from build123d import *

# Parameters (mm, degrees)
SKETCH1_R                                      = 44.45
BOSS_EXTRUDE1_DEPTH                            = 6.35
SKETCH2_R                                      = 13.5
CUT_EXTRUDE1_DEPTH                             = 65.131856359
CSK_FOR_0_FLAT_HEAD_MACHINE_SCREW1_D           = 1.778
CSK_FOR_0_FLAT_HEAD_MACHINE_SCREW1_CSINK_D     = 3.0226
CSK_FOR_0_FLAT_HEAD_MACHINE_SCREW1_CSINK_ANGLE = 82
CIRPATTERN1_COUNT                              = 8
SKETCH6_W                                      = 12.7
SKETCH6_H                                      = 25.4
BOSS_EXTRUDE2_DEPTH                            = 50.8
FILLET1_R                                      = 12.7
SKETCH7_R                                      = 6.35
CUT_EXTRUDE2_DEPTH                             = 106.111203019


with BuildPart() as part:
    # Sketch1 → Boss-Extrude1 (new, symmetric)
    with BuildSketch(Plane.XY):
        Circle(SKETCH1_R)
    extrude(amount=BOSS_EXTRUDE1_DEPTH, both=True)

    # Sketch2 → Cut-Extrude1 (cut, through all)
    with BuildSketch(Plane.XY.offset(6.35)):
        Circle(SKETCH2_R)
    extrude(amount=-CUT_EXTRUDE1_DEPTH, mode=Mode.SUBTRACT)

    # CSK for #0 Flat Head Machine Screw1 (through all)
    with Locations(Plane(origin=(-0.166965968, 41.999668122, 6.35), x_dir=(1, 0, 0), z_dir=(0, 0, 1))):
        with Locations((0, 0)):
            csk_for_0_flat_head_machine_screw1 = CounterSinkHole(CSK_FOR_0_FLAT_HEAD_MACHINE_SCREW1_D / 2, CSK_FOR_0_FLAT_HEAD_MACHINE_SCREW1_CSINK_D / 2, counter_sink_angle=CSK_FOR_0_FLAT_HEAD_MACHINE_SCREW1_CSINK_ANGLE)

    # CirPattern1: CSK for #0 Flat Head Machine Screw1 ×8 about axis
    cirpattern1_axis = Axis((0, 0, 0), (0, 0, 1))
    for i in range(1, CIRPATTERN1_COUNT):
        add(csk_for_0_flat_head_machine_screw1.rotate(cirpattern1_axis, i * 360 / CIRPATTERN1_COUNT), mode=Mode.SUBTRACT)

    # Sketch6 → Boss-Extrude2 (add)
    with BuildSketch(Plane.XY.offset(6.35)):
        with Locations((-25.4, 0)):
            Rectangle(SKETCH6_W, SKETCH6_H)
        with Locations((25.4, 0)):
            Rectangle(SKETCH6_W, SKETCH6_H)
    extrude(amount=BOSS_EXTRUDE2_DEPTH)

    # Fillet1
    fillet1_edges = [part.edges().sort_by_distance(p)[0] for p in [
        (-25.4, 12.7, 57.15),
        (-25.4, -12.7, 57.15),
        (25.4, -12.7, 57.15),
        (25.4, 12.7, 57.15),
    ]]
    fillet(fillet1_edges, radius=FILLET1_R - 0.0001)  # a hair under: the kernel refuses the full size

    # Sketch7 → Cut-Extrude2 (cut, through all)
    with BuildSketch(Plane(origin=(31.75, 0, 0), x_dir=(0, 0, -1), z_dir=(1, 0, 0))):
        with Locations((-44.45, 0)):
            Circle(SKETCH7_R)
    extrude(amount=-CUT_EXTRUDE2_DEPTH, mode=Mode.SUBTRACT)


solid = part.part
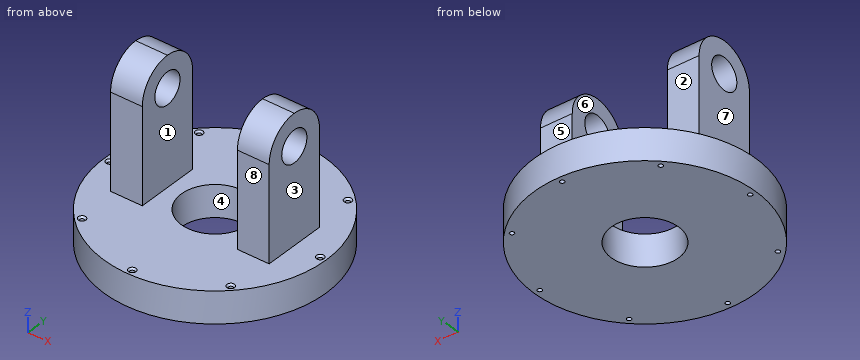
Geometry check sheet. Reference: the model listing, model coordinates, mm. Face numbers are marked on the shaded views. A direction names the side the tool comes from. Coordinates: 2 decimals unless noted, no trailing zeros. Order: outer loops, then holes, each group sorted by start corner. A loop starts at its lowest first (then second) coordinate and runs counter-clockwise, first axis right, second up. Notation, with made-up numbers: (54, 21) -> (108, 21) arc R30 ccw to (108, 46) -> close; hole circle Ø5 at (-6.75, -40). An arc over 180 degrees is marked (long way). Use a Markdown table: item, result. Add a question column.
1. Mould release check, pull along X, two halves, no side actions. Record for the marked faces 1, 2, 3 and 4: pulls with the +X half, pulls with the -X half, needs draft (parallel to the pull), parting line crosses it, or undercut.
2. Set-up check for the marked faces 5, 6, 7 and 8: record each of +Z, -Z, +X, -X, +Y, -Y from which the full face is reachable in a straight line by a thin tool's end or side.
3. Cross-section at D-D (y = 36.5). Enter the section's corners in (x, z), and give its area (3 significant figures).
4. Cross-section at A-A (z = 10). Enter the section's corners in (x, y), and give its area (3 significant figures).
5. Go/stop test with flat-tipped pins: pin 1 Ø2 at (x, y) = (29.58, 29.82) entering from +Z; pin 2 Ø6.5 at (x, z) = (-24, 17) entering from -Y; pin 3 Ø1.5 at (x, z) = (-20, 29) entering from +Y; pin 4 Ø7.5 at (y, z) = (0, 44.45) entering from -X. Record where each tip stops, or that it passes through.
6. Cross-section at C-C (y = 10). Enter the section's corners in (x, z), and give its area (3 significant figures).
7. Cross-section at B-B (x = -9). Enter the section's corners in (y, z).
8. Material ranges on L1, parallel to X at y = 12, z = 44; L2, parallel to Y at x = 0, z = 3.5; L3, parallel to Y at x = 25, z = 44, recorded low to high.
Filled sheet:
| question | item | result |
|---|---|---|
| 1 | face 1 | undercut |
| 1 | face 2 | needs draft |
| 1 | face 3 | pulls with the +X half |
| 1 | face 4 | undercut |
| 2 | face 5 | +Z, +X, -X, +Y |
| 2 | face 6 | +Z, +Y, -Y |
| 2 | face 7 | +Z, -X, +Y, -Y |
| 2 | face 8 | +Z, +X, -X, -Y |
| 3 | outline | (-25.37, -6.35) -> (25.37, -6.35) -> (25.37, 6.35) -> (-25.37, 6.35) -> close |
| 3 | area | 644 mm2 |
| 4 | outline | (-31.75, -12.7) -> (-19.05, -12.7) -> (-19.05, 12.7) -> (-31.75, 12.7) -> close; (19.05, -12.7) -> (31.75, -12.7) -> (31.75, 12.7) -> (19.05, 12.7) -> close |
| 4 | area | 645 mm2 |
| 5 | pin 1 | z = 5.77 |
| 5 | pin 2 | y = -12.7 |
| 5 | pin 3 | y = 12.7 |
| 5 | pin 4 | through |
| 6 | outline | (-43.31, -6.35) -> (-9.07, -6.35) -> (-9.07, 6.35) -> (-19.05, 6.35) -> (-19.05, 52.28) -> (-31.75, 52.28) -> (-31.75, 6.35) -> (-43.31, 6.35) -> close; (9.07, -6.35) -> (43.31, -6.35) -> (43.31, 6.35) -> (31.75, 6.35) -> (31.75, 52.28) -> (19.05, 52.28) -> (19.05, 6.35) -> (9.07, 6.35) -> close |
| 6 | area | 2,040 mm2 |
| 7 | outline | (-43.53, -6.35) -> (-10.06, -6.35) -> (-10.06, 6.35) -> (-43.53, 6.35) -> close; (10.06, -6.35) -> (43.53, -6.35) -> (43.53, 6.35) -> (10.06, 6.35) -> close |
| 8 | L1 | -31.75 to -19.05, 19.05 to 31.75 |
| 8 | L2 | -44.45 to -42.87, -41.13 to -13.5, 13.5 to 41.13, 42.87 to 44.45 |
| 8 | L3 | -12.7 to -6.33, 6.33 to 12.7 |
